Job drawing, mm, ordinate dimensions from the low corner. One solid piece. A direction names the side the tool comes from. Round coordinates to 2 decimals unless told otherwise and drop trailing zeros. Loops run counter-clockwise (first coordinate to the right, second up) from the corner with the lowest first, then second, coordinate; pieces in that order, holes last. Notation, with made-up numbers: M 12.25,70 L 32.25,70 A13 ccw 32.25,95 Z; hole C 81,-8 d10. An arc over 180 degrees is marked long. Use a Markdown table: item, result. Add a question column.
(1) Band-saw the part on C-C, the plane x = 51. Write the cut outline in (y, z).
(2) Wall check: L1, parallel to X at y = 33, z = 7.25; L2, parallel to Y at x = 6.5, z = 12; L3, parallel to X at y = 50, z = 12 (1 decimal). Give the ranges that are in metal, low to high.
(3) Flat gauge pins, fed straight in: P1, Ø1, axis at y = 24, z = 17, coming from the +X side; P2, Ø1.5, axis at x = 26.5, y = 12, coming from the -Z side; P3, Ø3, axis at y = 59, z = 18, coming from the -X side; P4, Ø2, axis at x = 23.5, z = 19.5, coming from the +Y side. Where does each tip first touch, or does it go through?
(4) Which spindle directions (+Z, -Z, +X, -X, +Y, -Y) get a long thin tool onto all of the face, cutting with end or side? Do the marked faces 5, 6 and 7. Say none if no direction does.
(5) Band-saw the part on B-B, the plane y = 49. Write the cut outline in (x, z) (1 decimal).
(6) Two-plate mould, pull along X, no slides. Class the marked faces 1, 2, 3 and 4: released by +X, released by -X, zero draft, split by the parting line, or undercut.
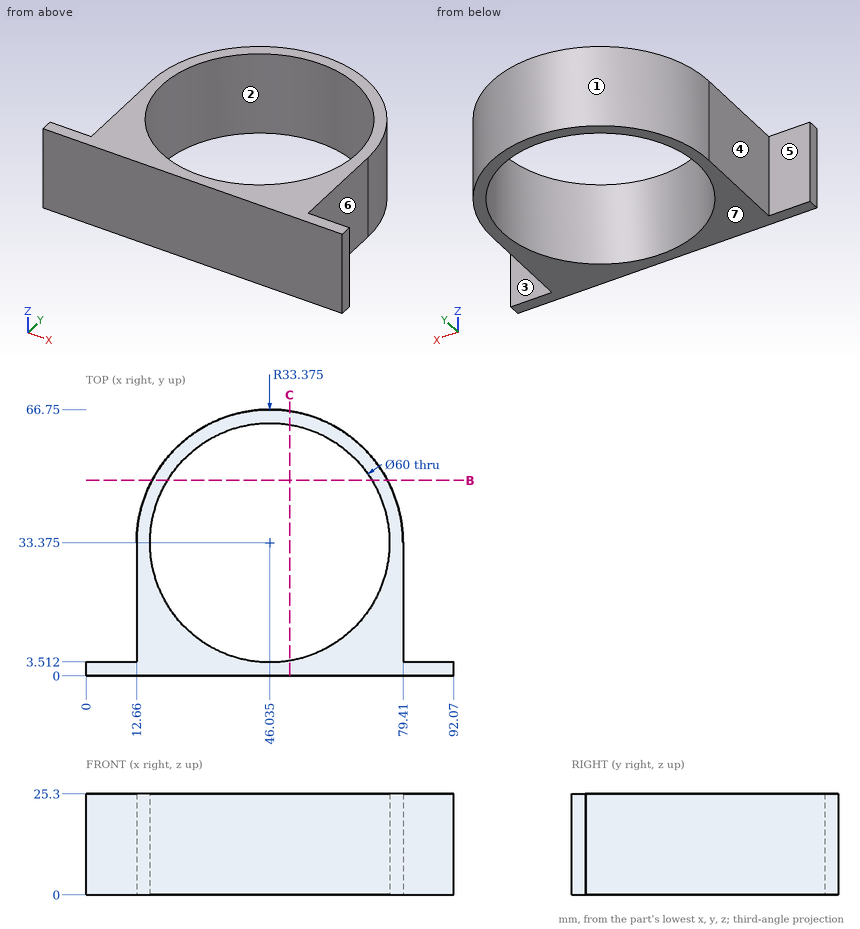
Return value:
| question | item | result |
|---|---|---|
| 1 | outline | M 0,0 L 3.79,0 L 3.79,25.3 L 0,25.3 Z; M 62.96,0 L 66.38,0 L 66.38,25.3 L 62.96,25.3 Z |
| 2 | L1 | 12.66 to 16.04, 76.03 to 79.41 |
| 2 | L2 | 0 to 3.51 |
| 2 | L3 | 17.1 to 21.1, 71 to 75 |
| 3 | P1 | x = 79.41 |
| 3 | P2 | through |
| 3 | P3 | x = 22.97 |
| 3 | P4 | y = 58.87 |
| 4 | face 5 | +Z, -Z, -X, +Y |
| 4 | face 6 | +Z, -Z, +X, +Y |
| 4 | face 7 | -Z, +X, -X, +Y, -Y |
| 5 | outline | M 16.5,0 L 20.4,0 L 20.4,25.3 L 16.5,25.3 Z; M 71.6,0 L 75.5,0 L 75.5,25.3 L 71.6,25.3 Z |
| 6 | face 1 | split by the parting line |
| 6 | face 2 | undercut |
| 6 | face 3 | zero draft |
| 6 | face 4 | released by -X |
